Could you check a few things on this model? Use its own coordinates, in mm. A direction names the side the tool comes from. Round coordinates to 2 decimals unless told otherwise and drop trailing zeros. Loops run counter-clockwise (first coordinate to the right, second up) from the corner with the lowest first, then second, coordinate; pieces in that order, holes last.
from build123d import *

# Parameters (mm, degrees)
SKETCH1_R               = 7.5
BOSS_EXTRUDE1_DEPTH     = 58
CUT_EXTRUDE1_DEPTH      = 90.381206078
CUT_EXTRUDE1_DEPTH_BACK = 90.381206078
CUT_EXTRUDE2_DEPTH      = 96.859271852
CUT_EXTRUDE2_DEPTH_BACK = 96.859271852
CUT_EXTRUDE3_DEPTH      = 107.60206377
CUT_EXTRUDE3_DEPTH_BACK = 107.60206377
SKETCH7_R               = 7
CUT_EXTRUDE6_DEPTH      = 12
CUT_EXTRUDE7_DEPTH      = 6


with BuildPart() as part:
    # Sketch1 → Boss-Extrude1 (new body)
    with BuildSketch(Plane.XY):
        with BuildLine():
            Line((0, 0), (-65, 0))
            Line((-65, 0), (-65, 24))
            ThreePointArc((-65, 24), (-48.33939444, 35.82575695), (-28.33939444, 40))
            Line((-28.33939444, 40), (0, 40))
            Line((0, 40), (15, 31.339745962))
            Line((15, 31.339745962), (15, 8.660254038))
            Line((15, 8.660254038), (0, 0))
        make_face()
        with Locations(Location((-31, 19, 0), (0, 0, 180))):
            Circle(SKETCH1_R, mode=Mode.SUBTRACT)
    extrude(amount=BOSS_EXTRUDE1_DEPTH)

    # Sketch3 → Cut-Extrude1 (cut, two sides: drawn at the far end of the back side and taken through both)
    with BuildSketch(Plane(origin=(0, 20, 0), x_dir=(1, 0, 0), z_dir=(0, 1, 0)).offset(-CUT_EXTRUDE1_DEPTH_BACK)):
        Polygon((-11, -44), (-11, -14), (-49, -14), (-49, -8), (-65, -8), (-65, -50), (-49, -50), (-49, -44), align=None)
    extrude(amount=CUT_EXTRUDE1_DEPTH + CUT_EXTRUDE1_DEPTH_BACK, mode=Mode.SUBTRACT)

    # Sketch6 → Cut-Extrude2 (cut, two sides: drawn at the far end of the back side and taken through both)
    with BuildSketch(Plane(origin=(0, 0, 0), x_dir=(1, 0, 0), z_dir=(0, 1, 0)).offset(-CUT_EXTRUDE2_DEPTH_BACK)):
        Polygon((0, 0), (15, -15), (15, 0), align=None)
        Polygon((15, -58), (15, -43), (0, -58), align=None)
    extrude(amount=CUT_EXTRUDE2_DEPTH + CUT_EXTRUDE2_DEPTH_BACK, mode=Mode.SUBTRACT)

    # Sketch7 → Cut-Extrude3 (cut, two sides: drawn at the far end of the back side and taken through both)
    with BuildSketch(Plane(origin=(15, 0, 0), x_dir=(0, 0, -1), z_dir=(1, 0, 0)).offset(-CUT_EXTRUDE3_DEPTH_BACK)):
        with Locations(Location((-29, 20, 0), (0, 0, 90))):
            Circle(SKETCH7_R)
    extrude(amount=CUT_EXTRUDE3_DEPTH + CUT_EXTRUDE3_DEPTH_BACK, mode=Mode.SUBTRACT)

    # Sketch8 → Cut-Extrude6 (cut)
    with BuildSketch(Plane.XY.offset(58)):
        with BuildLine():
            Line((-47, 34.224221872), (-47, 2))
            Line((-47, 2), (-2, 2))
            Line((-2, 2), (-2, 38))
            Line((-2, 38), (-28.33939444, 38))
            ThreePointArc((-28.33939444, 38), (-37.858778616, 37.046586751), (-47, 34.224221872))
        make_face()
    extrude(amount=-CUT_EXTRUDE6_DEPTH, mode=Mode.SUBTRACT)

    # Sketch16 → Cut-Extrude7 (cut)
    with BuildSketch(Plane.XY.offset(58)):
        with BuildLine():
            Line((-65, 21.1865019), (-65, 2))
            Line((-65, 2), (-47, 2))
            Line((-47, 2), (-47, 34.224221872))
            ThreePointArc((-47, 34.224221872), (-56.733711161, 28.718330483), (-65, 21.1865019))
        make_face()
    extrude(amount=-CUT_EXTRUDE7_DEPTH, mode=Mode.SUBTRACT)


solid = part.part
Item 1: For faces 5 (the cylindrical face through (-44.34, 37.37, 5.35)), 6 (the flat face through (-21, 20, 14)), 7 (the flat face through (-47, 18, 49)), which set-ups out of +Z, -Z, +X, -X, +Y, -Y let a thin tool reach every point of the face, with its end or its side?
Results list:
face 5: +Z, -Z, -X, +Y
face 6: -X, +Y, -Y
face 7: +Z
Item 2: Will these pins go through, and if not, where does the flat tip stop? pin 1 (19 mm diameter, centred on x = -27, y = 26.5, fed in from +Z); pin 2 (17 mm diameter, centred on x = -31, y = 19, fed in from -Z); pin 3 (1.8 mm diameter, centred on y = 11, z = 10, fed in from -X); pin 4 (9 mm diameter, centred on y = 30, z = 30, fed in from -X).
Results list:
pin 1: stops at z = 46
pin 2: stops at z = 0
pin 3: stops at x = -49
pin 4: stops at x = -11
Item 3: We'd pull the mould along X, two halves only. Please class faces 1 (the cylindrical face through (-37.727, 37.073, 52.084)), 2 (the flat face through (-65, 12, 4)), 3 (the flat face through (8, 20, 50)), 4 (the flat face through (-10, 0, 29)): released by +X, released by -X, zero draft, split by the parting line, or undercut.
Results list:
face 1: undercut
face 2: released by -X
face 3: released by +X
face 4: zero draft
Item 4: If we section it at A-A, the plane z = 29: Please give me the cut outline in (x, y), then the cut area to 3 significant figures.
Results list:
outline: (-11, 0) - (0, 0) - (15, 8.66) - (15, 13) - (-11, 13) - close; (-11, 27) - (15, 27) - (15, 31.34) - (0, 40) - (-11, 40) - close
area: 546 mm2
Item 5: If we section it at D-D, the plane x = -31: Please give me the cut outline in (y, z), then the cut area to 3 significant figures.
Results list:
outline: (0, 0) - (11.5, 0) - (11.5, 14) - (0, 14) - close; (0, 44) - (11.5, 44) - (11.5, 46) - (2, 46) - (2, 58) - (0, 58) - close; (26.5, 0) - (39.93, 0) - (39.93, 14) - (26.5, 14) - close; (26.5, 44) - (39.93, 44) - (39.93, 58) - (37.93, 58) - (37.93, 46) - (26.5, 46) - close
area: 447 mm2
Item 6: If we section it at B-B, the plane x = -10: Please give me the cut outline in (y, z), then the cut area to 3 significant figures.
Results list:
outline: (0, 0) - (40, 0) - (40, 58) - (38, 58) - (38, 46) - (2, 46) - (2, 58) - (0, 58) - close; hole circle Ø14 at (20, 29)
area: 1,730 mm2
Item 7: If we section it at C-C, the plane y = 19: Count the separate pieces of the cut face and the enclosed holes in it, then the cut area to 3 significant figures.
Results list:
separate pieces: 4
enclosed holes: 0
area: 1,350 mm2
Item 8: If I drill on line 1 along Z through (x, y) = (-43, 35); line 2 along Y through (x, z) = (-0.75, 29); line 3 along Z through (x, y) = (-14, 38.5), over which ranges is the centre line in solid material (lowest first)?
Results list:
line 1: z = 0 to 14, 44 to 46
line 2: y = 0 to 13, 27 to 40
line 3: z = 0 to 14, 44 to 58
